Source: CAD feature listing. Evaluate the final solid. Frame: model axes, mm. A direction names the side the tool comes from. Give positions to 0.01 mm unless a question says otherwise; leave off trailing zeros. Loops run counter-clockwise (first coordinate to the right, second up) from the corner with the lowest first, then second, coordinate; pieces in that order, holes last. Notation, with made-up numbers: M 12,12.5 L 25,12.5 A21 ccw 25,18.5 Z; hole C 12,27.5 d6. An arc over 180 degrees is marked long. Answer in a Markdown table with one row per item.
```python
from build123d import *

# Parameters (mm, degrees)
SKETCH_1_W               = 115
SKETCH_1_H               = 150
EXTRUDE_1_DEPTH          = 32
SKETCH_2_R               = 34
CUT_EXTRUDE_1_DEPTH      = 100.775999118
SKETCH_3_W               = 40
SKETCH_3_H               = 85
CUT_EXTRUDE_2_DEPTH      = 20
F_1_0MM_2_D              = 2.6
SKETCH_8_W               = 5
SKETCH_8_H               = 40
CUT_EXTRUDE_3_DEPTH      = 100.775999118
CUT_EXTRUDE_4_REACH      = 165.799
CUT_EXTRUDE_4_END_RADIUS = 34
SKETCH_9_W               = 22
SKETCH_9_H               = 20
CUT_EXTRUDE_5_REACH      = 142.975
FILLET_1_SIZE            = 8
F_1_0MM_4_AT_2_COUNT     = 2
F_1_0MM_4_AT_2_PITCH     = 15
F_1_0MM_3_D              = 2.6
F_1_0MM_3_DEPTH          = 7.5
F_1_0MM_3_TIP            = 0.781118805
CUT_EXTRUDE_7_DEPTH      = 20
F_1_0MM_5_REACH          = 142.975
F_1_0MM_5_BORE_R         = 1.65
F_1_0MM_6_D              = 2.7


with BuildPart() as part:
    # Sketch 1 → Extrude 1 (new body)
    with BuildSketch(Plane.XY):
        Rectangle(SKETCH_1_W, SKETCH_1_H)
    extrude(amount=EXTRUDE_1_DEPTH)

    # Sketch 2 → Cut-Extrude 1 (cut, through all)
    with BuildSketch(Plane.XY.offset(32)):
        with Locations((0, 32.5)):
            Circle(SKETCH_2_R)
    extrude(amount=-CUT_EXTRUDE_1_DEPTH, mode=Mode.SUBTRACT)

    # Sketch 3 → Cut-Extrude 2 (cut)
    with BuildSketch(Plane.XY.offset(32)):
        with Locations((-29.5, -24.5)):
            Rectangle(SKETCH_3_W, SKETCH_3_H)
    cut_extrude_2 = extrude(amount=-CUT_EXTRUDE_2_DEPTH, mode=Mode.SUBTRACT)

    # Mirror 1: Cut-Extrude 2 across plane
    add(cut_extrude_2.mirror(Plane(origin=(0, 0, 0), x_dir=(0, 0, 1), z_dir=(1, 0, 0))), mode=Mode.SUBTRACT)

    # 1.0mm _2 (through all)
    with Locations(Plane(origin=(0, 0, 0), x_dir=(-1, 0, 0), z_dir=(0, 0, -1))):
        with Locations((47.5, -8), (47.5, -63), (-47.5, -8), (-47.5, -63)):
            Hole(F_1_0MM_2_D / 2)

    # Sketch 8 → Cut-Extrude 3 (cut, through all)
    with BuildSketch(Plane.XY.offset(32)):
        with Locations((-50, 55)):
            Rectangle(SKETCH_8_W, SKETCH_8_H)
    cut_extrude_3 = extrude(amount=-CUT_EXTRUDE_3_DEPTH, mode=Mode.SUBTRACT)

    # Mirror 2: Cut-Extrude 3 across plane
    add(cut_extrude_3.mirror(Plane(origin=(0, 0, 0), x_dir=(0, 0, 1), z_dir=(1, 0, 0))), mode=Mode.SUBTRACT)

    # Cut-Extrude 4: up to this cylinder (the profile starts outside it)
    cut_extrude_4_end = Plane(origin=(0, 32.5, 22), z_dir=(0, 0, 1)) * Cylinder(CUT_EXTRUDE_4_END_RADIUS, 400.598, mode=Mode.PRIVATE)
    # Sketch 9 → Cut-Extrude 4 (cut, up to the surface)
    with BuildSketch(Plane(origin=(0, 75, 0), x_dir=(1, 0, 0), z_dir=(0, 1, 0)), mode=Mode.PRIVATE) as cut_extrude_4_sk1:
        with Locations((0, -22)):
            Rectangle(SKETCH_9_W, SKETCH_9_H)
    cut_extrude_4_tool1 = extrude(cut_extrude_4_sk1.sketch, amount=-CUT_EXTRUDE_4_REACH, mode=Mode.PRIVATE) - cut_extrude_4_end
    add(cut_extrude_4_tool1.solids().sort_by_distance((0, 75, 22))[0], mode=Mode.SUBTRACT)

    # Sketch 11 → Cut-Extrude 5 (cut, up to next)
    with BuildSketch(Plane(origin=(57.5, 0, 0), x_dir=(0, 0, -1), z_dir=(1, 0, 0)), mode=Mode.PRIVATE) as cut_extrude_5_sk1:
        with BuildLine():
            Line((-13.9, 65), (-13.9, 40))
            ThreePointArc((-13.9, 40), (-16, 37.9), (-18.1, 40))
            Line((-18.1, 40), (-18.1, 65))
            ThreePointArc((-18.1, 65), (-16, 67.1), (-13.9, 65))
        make_face()
    cut_extrude_5_tool1 = extrude(cut_extrude_5_sk1.sketch, amount=-CUT_EXTRUDE_5_REACH, mode=Mode.PRIVATE) & part.part
    cut_extrude_5 = cut_extrude_5_tool1.solids().sort_by_distance((57.5, 52.5, 16))[0]
    add(cut_extrude_5, mode=Mode.SUBTRACT)

    # Mirror 3: Cut-Extrude 5 across plane
    add(cut_extrude_5.mirror(Plane(origin=(0, 0, 0), x_dir=(0, 0, 1), z_dir=(1, 0, 0))), mode=Mode.SUBTRACT)

    # Fillet 1
    # a fillet whose section is not a circle: 8 mm, written as the material it takes off along each edge
    with BuildSketch(Plane(origin=(-32.5, 75, 32), x_dir=(0, -1, 0), z_dir=(-1, 0, 0))) as fillet_1_piece_1_section:
        with BuildLine():
            Bezier((FILLET_1_SIZE, 0), (0, 0), (0, -FILLET_1_SIZE), weights=[1, 1, 1])
            Line((0, -FILLET_1_SIZE), (0, 0))
            Line((0, 0), (FILLET_1_SIZE, 0))
        make_face()
    fillet_1_piece_1 = extrude(amount=45, mode=Mode.PRIVATE)
    fillet_1_piece_1 = split(fillet_1_piece_1, bisect_by=Plane(origin=(-47.5, 75, 32), z_dir=(-1, 0, 0)), keep=Keep.TOP, mode=Mode.PRIVATE)
    add(fillet_1_piece_1, mode=Mode.SUBTRACT)
    with BuildSketch(Plane(origin=(-32.5, 75, 0), x_dir=(0, -1, 0), z_dir=(-1, 0, 0))) as fillet_1_piece_2_section:
        with BuildLine():
            Bezier((FILLET_1_SIZE, 0), (0, 0), (0, FILLET_1_SIZE), weights=[1, 1, 1])
            Line((0, FILLET_1_SIZE), (0, 0))
            Line((0, 0), (FILLET_1_SIZE, 0))
        make_face()
    fillet_1_piece_2 = extrude(amount=45, mode=Mode.PRIVATE)
    fillet_1_piece_2 = split(fillet_1_piece_2, bisect_by=Plane(origin=(-47.5, 75, 0), z_dir=(-1, 0, 0)), keep=Keep.TOP, mode=Mode.PRIVATE)
    add(fillet_1_piece_2, mode=Mode.SUBTRACT)
    with BuildSketch(Plane(origin=(77.5, 75, 0), x_dir=(0, -1, 0), z_dir=(-1, 0, 0))) as fillet_1_piece_3:
        with BuildLine():
            Bezier((FILLET_1_SIZE, 0), (0, 0), (0, FILLET_1_SIZE), weights=[1, 1, 1])
            Line((0, FILLET_1_SIZE), (0, 0))
            Line((0, 0), (FILLET_1_SIZE, 0))
        make_face()
    extrude(amount=25, mode=Mode.SUBTRACT)
    with BuildSketch(Plane(origin=(77.5, 75, 32), x_dir=(0, -1, 0), z_dir=(-1, 0, 0))) as fillet_1_piece_4:
        with BuildLine():
            Bezier((FILLET_1_SIZE, 0), (0, 0), (0, -FILLET_1_SIZE), weights=[1, 1, 1])
            Line((0, -FILLET_1_SIZE), (0, 0))
            Line((0, 0), (FILLET_1_SIZE, 0))
        make_face()
    extrude(amount=25, mode=Mode.SUBTRACT)

    # Sketch 13 → 1.0mm _4 (revolve, cut)
    with BuildSketch(Plane(origin=(-37.5, 75, 15), x_dir=(0, 0, 1), z_dir=(1, 0, 0))):
        Polygon((0, 0), (0, 16.59228064), (2.65, 15), (2.65, 0), align=None)
    f_1_0mm_4 = revolve(axis=Axis((-37.5, 81.35, 15), (0, -1, 0)), mode=Mode.SUBTRACT)

    # 1.0mm _4 at 2: 1.0mm _4 ×2
    with Locations(*[(i * F_1_0MM_4_AT_2_PITCH, 0, 0) for i in range(1, F_1_0MM_4_AT_2_COUNT)]):
        add(f_1_0mm_4, mode=Mode.SUBTRACT)

    # Mirror 4: 1.0mm _4 across plane
    add(f_1_0mm_4.mirror(Plane(origin=(0, 0, 0), x_dir=(0, 0, 1), z_dir=(1, 0, 0))), mode=Mode.SUBTRACT)

    # Mirror 4 copy 1 sketch → Mirror 4 copy 1 (revolve, cut)
    with BuildSketch(Plane(origin=(22.5, 75, 15), x_dir=(0, 0, 1), z_dir=(-1, 0, 0))):
        Polygon((0, 0), (0, -16.59228064), (2.65, -15), (2.65, 0), align=None)
    revolve(axis=Axis((22.5, 81.35, 15), (0, 1, 0)), mode=Mode.SUBTRACT)

    # 1.0mm _3
    with Locations(Plane.XY.offset(32)):
        with Locations((-52.5, -70), (51.464741732, -70), (-42.5, 70), (-42.5, 30), (42.5, 70), (42.5, 30)):
            Hole(F_1_0MM_3_D / 2, depth=F_1_0MM_3_DEPTH)
            with Locations((0, 0, -(F_1_0MM_3_DEPTH + F_1_0MM_3_TIP / 2))):  # 118° drill point
                Cone(0, F_1_0MM_3_D / 2, F_1_0MM_3_TIP, mode=Mode.SUBTRACT)

    # Sketch 17 → Cut-Extrude 7 (cut)
    with BuildSketch(Plane.XY.offset(32)):
        with BuildLine():
            Line((-49.5, 18), (-34, 32.5))
            ThreePointArc((-34, 32.5), (-33.178333694, 25.070452685), (-30.753048629, 18))
            Line((-30.753048629, 18), (-49.5, 18))
        make_face()
    cut_extrude_7 = extrude(amount=-CUT_EXTRUDE_7_DEPTH, mode=Mode.SUBTRACT)

    # 1.0mm _5 bore → 1.0mm _5 (cut, up to next)
    with BuildSketch(Plane.ZY.offset(57.5), mode=Mode.PRIVATE) as f_1_0mm_5_sk1:
        with Locations((16, -60)):
            Circle(F_1_0MM_5_BORE_R)
    f_1_0mm_5_tool1 = extrude(f_1_0mm_5_sk1.sketch, amount=-F_1_0MM_5_REACH, mode=Mode.PRIVATE) & part.part
    # 1.0mm _5 bore → 1.0mm _5 (cut, up to next)
    with BuildSketch(Plane.ZY.offset(57.5), mode=Mode.PRIVATE) as f_1_0mm_5_sk2:
        with Locations((16, -45)):
            Circle(F_1_0MM_5_BORE_R)
    f_1_0mm_5_tool2 = extrude(f_1_0mm_5_sk2.sketch, amount=-F_1_0MM_5_REACH, mode=Mode.PRIVATE) & part.part
    # 1.0mm _5 bore → 1.0mm _5 (cut, up to next)
    with BuildSketch(Plane.ZY.offset(57.5), mode=Mode.PRIVATE) as f_1_0mm_5_sk3:
        with Locations((16, -30)):
            Circle(F_1_0MM_5_BORE_R)
    f_1_0mm_5_tool3 = extrude(f_1_0mm_5_sk3.sketch, amount=-F_1_0MM_5_REACH, mode=Mode.PRIVATE) & part.part
    f_1_0mm_5_1 = f_1_0mm_5_tool1.solids().sort_by_distance((-57.5, -60, 16))[0]
    add(f_1_0mm_5_1, mode=Mode.SUBTRACT)
    f_1_0mm_5_2 = f_1_0mm_5_tool2.solids().sort_by_distance((-57.5, -45, 16))[0]
    add(f_1_0mm_5_2, mode=Mode.SUBTRACT)
    f_1_0mm_5_3 = f_1_0mm_5_tool3.solids().sort_by_distance((-57.5, -30, 16))[0]
    add(f_1_0mm_5_3, mode=Mode.SUBTRACT)
    f_1_0mm_5 = f_1_0mm_5_1 + f_1_0mm_5_2 + f_1_0mm_5_3  # 1.0mm _5 as one shape, for the pattern or mirror that repeats it

    # Mirror 5: 1.0mm _5 across plane
    add(f_1_0mm_5.mirror(Plane(origin=(0, 0, 0), x_dir=(0, 0, 1), z_dir=(1, 0, 0))), mode=Mode.SUBTRACT)

    # Mirror 6: Cut-Extrude 7 across plane
    add(cut_extrude_7.mirror(Plane(origin=(0, 0, 0), x_dir=(0, 0, 1), z_dir=(1, 0, 0))), mode=Mode.SUBTRACT)

    # 1.0mm _6 (through all)
    with Locations(Plane(origin=(0, 0, 0), x_dir=(-1, 0, 0), z_dir=(0, 0, -1))):
        with Locations((-29, 70), (-29, 5), (29, 70), (29, 5)):
            Hole(F_1_0MM_6_D / 2)


solid = part.part
```
Q1. Reachability of faces 1 (the cylindrical face through (-53.56, -28.61, 16.89)), 2 (the flat face through (49.5, -25, 22)), 3 (the flat face through (11, 70, 22)) from +Z, -Z, +X, -X, +Y, -Y: full face, straight path, thin tool, end or side. Return the list, or none.
Values follow:
| item | result |
|---|---|
| face 1 | -X |
| face 2 | +Z |
| face 3 | +Z, +Y |
Q2. Section query B-B (y = -45). Output: boundary loops of the cut face in (x, z).
Values follow:
| item | result |
|---|---|
| outline | M -57.5,0 L 57.5,0 L 57.5,14.35 L 49.5,14.35 L 49.5,12 L 9.5,12 L 9.5,32 L -9.5,32 L -9.5,12 L -49.5,12 L -49.5,14.35 L -57.5,14.35 Z; M -57.5,17.65 L -49.5,17.65 L -49.5,32 L -57.5,32 Z; M 49.5,17.65 L 57.5,17.65 L 57.5,32 L 49.5,32 Z |
Q3. Mould query, pull axis Y, two halves, no side actions, for faces 4 (the flat face through (-50, 35, 16)), 5 (the flat face through (-52.5, 55, 13)), 6 (the cylindrical face through (-55, 37.9, 16)). Classes: +Y half, -Y half, draft (parallel to the pull), parting line (faces both ways), or undercut.
Values follow:
| item | result |
|---|---|
| face 4 | +Y half |
| face 5 | draft |
| face 6 | undercut |
Q4. Section query A-A (x = 0). Output: boundary loops of the cut face in (y, z), plus the area to 3 significant figures.
Values follow:
| item | result |
|---|---|
| outline | M -75,0 L -1.5,0 L -1.5,32 L -75,32 Z; M 66.5,0 L 75,0 L 75,12 L 66.5,12 Z |
| area | 2,450 mm^2 |
Q5. Section query C-C (y = 15). Output: boundary loops of the cut face in (x, z), plus the area to 3 significant figures.
Values follow:
| item | result |
|---|---|
| outline | M -57.5,0 L -29.15,0 L -29.15,12 L -49.5,12 L -49.5,32 L -57.5,32 Z; M 29.15,0 L 57.5,0 L 57.5,32 L 49.5,32 L 49.5,12 L 29.15,12 Z |
| area | 1,000 mm^2 |
Q6. Contact query for flat-ended pins moving along their axis: pin 1 Ø12 at (x, y) = (-25.5, -8) entering from +Z; pin 2 Ø2 at (x, y) = (42.5, 70) entering from +Z; pin 3 Ø2 at (y, z) = (56, 15) entering from +X. Output: stop coordinate, or through.
Values follow:
| item | result |
|---|---|
| pin 1 | z = 12 |
| pin 2 | z = 24.32 |
| pin 3 | x = 47.5 |
Q7. Ray query, probe 1 along Y at (x, z) = (55.5, 16); probe 2 along X at (y, z) = (-11.5, 29.5); probe 3 along Y at (x, z) = (-42, 30.5). Return the intervals inside material, ascending. Write a range as from..to.
Values follow:
| item | result |
|---|---|
| probe 1 | -75..-61.65, -58.35..-46.65, -43.35..-31.65, -28.35..37.9, 67.1..75 |
| probe 2 | -57.5..-49.5, -9.5..9.5, 49.5..57.5 |
| probe 3 | -75..-67, 25.02..28.8, 31.2..68.8, 71.2..75 |
Q8. Section query D-D (z = 26.5). Give the number of separate pieces and of enclosed holes in the cut face, plus the area to 3 significant figures.
Values follow:
| item | result |
|---|---|
| separate pieces | 1 |
| enclosed holes | 8 |
| area | 6,420 mm^2 |
